Input: part model. Units: mm. Frame: model coordinates. A direction names the side the tool comes from. Round coordinates to 2 decimals unless told otherwise and drop trailing zeros. Write each loop counter-clockwise with the first axis right and the second up, starting at its lowest first coordinate (ties: lowest second). Pieces come first, ordered by that corner, then holes. Notation, with made-up numbers: M 86.5,-32.5 L 136.5,-32.5 A22 ccw 136.5,-8.5 Z; hole C 58.25,63.5 d6. An arc over 180 degrees is marked long. Write each question's results on one line, items separated by ' | '. Start each with the question number.
```python
from build123d import *

# Parameters (mm, degrees)
SKICA1_W                 = 50
SKICA1_H                 = 10
P_IDAT_VYSUNUT_M1_DEPTH  = 8
SKICA2_R                 = 1.65
ODEBRAT_VYSUNUT_M1_DEPTH = 52.613951602
ZAOBLIT2_R               = 5
SKICA4_R                 = 1.65
ODEBRAT_VYSUNUT_M2_DEPTH = 10
ODEBRAT_VYSUNUT_M3_DEPTH = 2.5
SKICA6_R                 = 3
ODEBRAT_VYSUNUT_M4_DEPTH = 2.5
SKICA7_W                 = 10
SKICA7_H                 = 10
P_IDAT_VYSUNUT_M2_DEPTH  = 36
SKICA8_W                 = 50
SKICA8_H                 = 10
P_IDAT_VYSUNUT_M3_DEPTH  = 8
ZAOBLIT3_R               = 5
ODEBRAT_START            = -8
SKICA9_R                 = 1.65
ODEBRAT_VYSUNUT_M5_DEPTH = 8
SKICA10_R                = 2.75
ODEBRAT_VYSUNUT_M6_DEPTH = 2.5
ODEBRAT_VYSUNUT_M7_DEPTH = 2.5
ODEBRAT_START_2          = -36
SKICA12_R                = 1.65
ODEBRAT_VYSUNUT_M8_DEPTH = 36


with BuildPart() as part:
    # Skica1 → Přidat vysunutím1 (new body)
    with BuildSketch(Plane.XY):
        with Locations((25, 5)):
            Rectangle(SKICA1_W, SKICA1_H)
    extrude(amount=P_IDAT_VYSUNUT_M1_DEPTH)

    # Skica2 → Odebrat vysunutím1 (cut, through all)
    with BuildSketch(Plane.XY.offset(8)):
        with Locations((5, 5)):
            Circle(SKICA2_R)
        with Locations((45, 5)):
            Circle(SKICA2_R)
    extrude(amount=-ODEBRAT_VYSUNUT_M1_DEPTH, mode=Mode.SUBTRACT)

    # Zaoblit2
    zaoblit2_edges = [part.edges().sort_by_distance(p)[0] for p in [
        (50, 0, 4),
        (50, 10, 4),
        (0, 0, 4),
        (0, 10, 4),
    ]]
    fillet(zaoblit2_edges, radius=ZAOBLIT2_R - 0.0001)  # a hair under: the kernel refuses the full size

    # Skica4 → Odebrat vysunutím2 (cut)
    with BuildSketch(Plane.XY.offset(8)):
        with Locations((25, 5)):
            Circle(SKICA4_R)
    extrude(amount=-ODEBRAT_VYSUNUT_M2_DEPTH, mode=Mode.SUBTRACT)

    # Skica5 → Odebrat vysunutím3 (cut)
    with BuildSketch(Plane(origin=(0, 0, 0), x_dir=(-1, 0, 0), z_dir=(0, 0, -1))):
        Polygon((-1.824573519, 5), (-3.41228676, 7.75), (-6.58771324, 7.75), (-8.175426481, 5), (-6.58771324, 2.25), (-3.41228676, 2.25), align=None)
    extrude(amount=-ODEBRAT_VYSUNUT_M3_DEPTH, mode=Mode.SUBTRACT)

    # Skica6 → Odebrat vysunutím4 (cut)
    with BuildSketch(Plane.XY.offset(8)):
        with Locations((45, 5)):
            Circle(SKICA6_R)
    extrude(amount=-ODEBRAT_VYSUNUT_M4_DEPTH, mode=Mode.SUBTRACT)

    # Skica7 → Přidat vysunutím2 (add)
    with BuildSketch(Plane(origin=(0, 0, 0), x_dir=(-1, 0, 0), z_dir=(0, 0, -1))):
        with Locations((-15, 5)):
            Rectangle(SKICA7_W, SKICA7_H)
    extrude(amount=P_IDAT_VYSUNUT_M2_DEPTH)

    # Skica8 → Přidat vysunutím3 (add)
    with BuildSketch(Plane(origin=(0, 0, -36), x_dir=(-1, 0, 0), z_dir=(0, 0, -1))):
        with Locations((-25, 5)):
            Rectangle(SKICA8_W, SKICA8_H)
    extrude(amount=P_IDAT_VYSUNUT_M3_DEPTH)

    # Zaoblit3
    zaoblit3_edges = [part.edges().sort_by_distance(p)[0] for p in [
        (0, 0, -40),
        (0, 10, -40),
        (50, 0, -40),
        (50, 10, -40),
    ]]
    fillet(zaoblit3_edges, radius=ZAOBLIT3_R - 0.0001)  # a hair under: the kernel refuses the full size

    # Skica9 → Odebrat vysunutím5 (cut)
    with BuildSketch(Plane(origin=(0, 0, -44), x_dir=(-1, 0, 0), z_dir=(0, 0, -1)).offset(ODEBRAT_START)):
        with Locations(Location((-45, 5, 0), (0, 0, 180))):
            Circle(SKICA9_R)
        with Locations(Location((-5, 5, 0), (0, 0, 180))):
            Circle(SKICA9_R)
    extrude(amount=ODEBRAT_VYSUNUT_M5_DEPTH, mode=Mode.SUBTRACT)

    # Skica10 → Odebrat vysunutím6 (cut)
    with BuildSketch(Plane(origin=(0, 0, -44), x_dir=(-1, 0, 0), z_dir=(0, 0, -1))):
        with Locations((-45, 5)):
            Circle(SKICA10_R)
    extrude(amount=-ODEBRAT_VYSUNUT_M6_DEPTH, mode=Mode.SUBTRACT)

    # Skica11 → Odebrat vysunutím7 (cut)
    with BuildSketch(Plane.XY.offset(-36)):
        Polygon((1.824573519, 5), (3.41228676, 2.25), (6.58771324, 2.25), (8.175426481, 5), (6.58771324, 7.75), (3.41228676, 7.75), align=None)
    extrude(amount=-ODEBRAT_VYSUNUT_M7_DEPTH, mode=Mode.SUBTRACT)

    # Skica12 → Odebrat vysunutím8 (cut)
    with BuildSketch(Plane(origin=(0, 0, -44), x_dir=(-1, 0, 0), z_dir=(0, 0, -1)).offset(ODEBRAT_START_2)):
        with Locations(Location((-25, 5, 0), (0, 0, 180))):
            Circle(SKICA12_R)
    extrude(amount=ODEBRAT_VYSUNUT_M8_DEPTH, mode=Mode.SUBTRACT)


solid = part.part
```
1. Access query for faces 4 (the face through (7.2, 2.8, 0)), 5 (the face through (47.747, 5.121, -42.768)), 6 (the face through (3.6, 6.3, 2.5)), 7 (the face through (20, 5, -18)), 8 (the face through (46.3, 3.7, 5.5)). Directions: +Z, -Z, +X, -X, +Y, -Y. A direction counts if a zero-diameter tool reaches every point of the face in a straight line with its end or side. Return the directions, or none.
2. Contact query for flat-ended pins moving along their axis: P1, Ø1, axis at y = 4, z = -4.5, coming from the +X side; P2, Ø6, axis at y = 4, z = -21.5, coming from the -X side. Output: stop coordinate, or through.
3. Draft query along X for faces 1 (the face through (43, 5, -41.5)), 2 (the face through (25, 7, -44)), 3 (the face through (10, 5, -18)). Return one class per face: +X half, -X half, draft (parallel to the pull), parting line (faces both ways), or undercut.
4. Cut plane A-A on x = 25. Output: boundary loops of the cut face in (y, z), and give its area (3 significant figures).
5. Cut plane B-B on z = -37. Give the number of separate pieces and of enclosed holes in the cut face, and give its area (3 significant figures).
6. Line query: L1, parallel to Z at x = 24, y = 7.75; L2, parallel to Y at x = 6, z = 1; L3, parallel to Z at x = 46.5, y = 7. Output: solid intervals per line, ascending. Write a range as from..to.
7. Cut plane C-C on x = 39. Output: boundary loops of the cut face in (y, z), and give its area (3 significant figures).
8. Cut plane D-D on z = -5. Output: boundary loops of the cut face in (x, y), and give its area (3 significant figures).
Answers follow:
1) face 4: -X, +Y, -Y | face 5: -Z | face 6: none | face 7: +X, +Y, -Y | face 8: +Z
2) P1: stops at x = 20 | P2: stops at x = 10
3) face 1: undercut | face 2: draft | face 3: -X half
4) outline: M 0,-44 L 3.35,-44 L 3.35,-36 L 0,-36 Z; M 0,0 L 3.35,0 L 3.35,8 L 0,8 Z; M 6.65,-44 L 10,-44 L 10,-36 L 6.65,-36 Z; M 6.65,0 L 10,0 L 10,8 L 6.65,8 Z | area: 107 mm2
5) separate pieces: 1 | enclosed holes: 3 | area: 435 mm2
6) L1: z = -44..-36, 0..8 | L2: y = 0..2.25, 7.75..10 | L3: z = -41.5..-36, 0..5.5
7) outline: M 0,-44 L 10,-44 L 10,-36 L 0,-36 Z; M 0,0 L 10,0 L 10,8 L 0,8 Z | area: 160 mm2
8) outline: M 10,0 L 20,0 L 20,10 L 10,10 Z | area: 100 mm2
